```python
from build123d import *

# Parameters (mm, degrees)
ESBO_O1_W                = 53
ESBO_O1_H                = 53
RESSALTO_EXTRUS_O1_DEPTH = 3
ESBO_O3_R                = 1.3
ESBO_O3_W                = 1.2
ESBO_O3_H                = 10
CORTE_EXTRUS_O1_DEPTH    = 38.596542394
ESBO_O4_W                = 1.55
ESBO_O4_H                = 7.65
ESBO_O4_W_2              = 7.65
ESBO_O4_H_2              = 1.55
CORTE_EXTRUS_O2_DEPTH    = 10
FILETE1_R                = 15
ESBO_O5_R                = 1
CORTE_EXTRUS_O3_DEPTH    = 38.596542394


with BuildPart() as part:
    # Esboço1 → Ressalto-extrusão1 (new body)
    with BuildSketch(Plane(origin=(0, 0, 0), x_dir=(1, 0, 0), z_dir=(0, 1, 0))):
        Rectangle(ESBO_O1_W, ESBO_O1_H)
    extrude(amount=RESSALTO_EXTRUS_O1_DEPTH)

    # Esboço3 → Corte-extrusão1 (cut, through all)
    with BuildSketch(Plane(origin=(0, 3, 0), x_dir=(1, 0, 0), z_dir=(0, 1, 0))):
        with Locations(Location((0, 0, 0), (0, 0, 270))):
            Circle(ESBO_O3_R)
        with Locations((-4.4, 0)):
            Rectangle(ESBO_O3_W, ESBO_O3_H)
        with Locations((4.4, 0)):
            Rectangle(ESBO_O3_W, ESBO_O3_H)
    extrude(amount=-CORTE_EXTRUS_O1_DEPTH, mode=Mode.SUBTRACT)

    # Esboço4 → Corte-extrusão2 (cut)
    with BuildSketch(Plane(origin=(0, 3, 0), x_dir=(-1, 0, 0), z_dir=(0, 1, 0))):
        with Locations((-7.725, -9.675)):
            Rectangle(ESBO_O4_W, ESBO_O4_H)
        with Locations((-9.675, 7.725)):
            Rectangle(ESBO_O4_W_2, ESBO_O4_H_2)
        with Locations((7.725, 9.675)):
            Rectangle(ESBO_O4_W, ESBO_O4_H)
        with Locations((9.675, -7.725)):
            Rectangle(ESBO_O4_W_2, ESBO_O4_H_2)
    extrude(amount=-CORTE_EXTRUS_O2_DEPTH, mode=Mode.SUBTRACT)

    # Filete1
    filete1_edges = [part.edges().sort_by_distance(p)[0] for p in [
        (26.5, 1.5, 26.5),
        (-26.5, 1.5, 26.5),
        (-26.5, 1.5, -26.5),
        (26.5, 1.5, -26.5),
    ]]
    fillet(filete1_edges, radius=FILETE1_R)

    # Esboço5 → Corte-extrusão3 (cut, through all)
    with BuildSketch(Plane(origin=(0, 3, 0), x_dir=(1, 0, 0), z_dir=(0, 1, 0))):
        with Locations(Location((-15.742640687, -21.399494937, 0), (0, 0, 270))):
            Circle(ESBO_O5_R)
        with Locations(Location((15.742640687, 21.399494937, 0), (0, 0, 270))):
            Circle(ESBO_O5_R)
        with BuildLine():
            Line((19.566648228, -3.32990767), (14.283511733, -3.32990767))
            ThreePointArc((14.283511733, -3.32990767), (10.953604064, 0), (14.283511733, 3.32990767))
            Line((14.283511733, 3.32990767), (19.566648228, 3.32990767))
            ThreePointArc((19.566648228, 3.32990767), (22.896555897, 0), (19.566648228, -3.32990767))
        make_face()
        with BuildLine():
            Line((-3.32990767, -19.566648228), (-3.32990767, -14.283511733))
            ThreePointArc((-3.32990767, -14.283511733), (0, -10.953604064), (3.32990767, -14.283511733))
            Line((3.32990767, -14.283511733), (3.32990767, -19.566648228))
            ThreePointArc((3.32990767, -19.566648228), (0, -22.896555897), (-3.32990767, -19.566648228))
        make_face()
        with BuildLine():
            Line((-19.566648228, 3.32990767), (-14.283511733, 3.32990767))
            ThreePointArc((-14.283511733, 3.32990767), (-10.953604064, 0), (-14.283511733, -3.32990767))
            Line((-14.283511733, -3.32990767), (-19.566648228, -3.32990767))
            ThreePointArc((-19.566648228, -3.32990767), (-22.896555897, 0), (-19.566648228, 3.32990767))
        make_face()
        with BuildLine():
            Line((3.32990767, 19.566648228), (3.32990767, 14.283511733))
            ThreePointArc((3.32990767, 14.283511733), (0, 10.953604064), (-3.32990767, 14.283511733))
            Line((-3.32990767, 14.283511733), (-3.32990767, 19.566648228))
            ThreePointArc((-3.32990767, 19.566648228), (0, 22.896555897), (3.32990767, 19.566648228))
        make_face()
    extrude(amount=-CORTE_EXTRUS_O3_DEPTH, mode=Mode.SUBTRACT)


solid = part.part
```
Input: part model. Units: mm. Frame: model coordinates. Round coordinates to 2 decimals unless told otherwise and drop trailing zeros. Loops run counter-clockwise (first coordinate to the right, second up) from the corner with the lowest first, then second, coordinate; pieces in that order, holes last. Notation, with made-up numbers: M 13.5,26.5 L 54.5,26.5 A20 ccw 54.5,42.5 Z; hole C 12,-2 d2. An arc over 180 degrees is marked long. Answer in a Markdown table with one row per item. Add a question column.
1. Contact query for flat-ended pins moving along their axis: pin 1 (0.9 mm diameter, centred on x = -17.5, y = 1.5, fed in from +Z); pin 2 (1.5 mm diameter, centred on x = -17, y = 2, fed in from -Z); pin 3 (1.5 mm diameter, centred on y = 2, z = -18, fed in from +X). Output: stop coordinate, or through.
2. Mould query, pull axis X, two halves, no side actions, for faces 1 (the face through (-8, 2, 13.5)), 2 (the face through (0, 1, 26.5)), 3 (the face through (21.99, 1.52, -22.22)), 4 (the face through (-22.22, 1.52, -21.99)). Classes: released by +X, released by -X, zero draft, split by the parting line, or undercut.
3. Section C-C (y = 2.35). Give the number of separate pieces and of enclosed holes in the cut face, and give its area (3 significant figures).
4. Section B-B (x = 0). Output: boundary loops of the cut face in (y, z).
5. Ray query, probe 1 along X at (y, z) = (2.5, 0); probe 2 along Z at (x, y) = (-6, 2.45); probe 3 along X at (y, z) = (0.4, 12). Return the intervals inside material, ascending.
6. Section A-A (z = 0). Output: boundary loops of the cut face in (x, y), and give its area (3 significant figures).
Values follow:
| question | item | result |
|---|---|---|
| 1 | pin 1 | z = 25.44 |
| 1 | pin 2 | z = -25.73 |
| 1 | pin 3 | x = 25.35 |
| 2 | face 1 | undercut |
| 2 | face 2 | zero draft |
| 2 | face 3 | released by +X |
| 2 | face 4 | released by -X |
| 3 | separate pieces | 1 |
| 3 | enclosed holes | 13 |
| 3 | area | 2,250 mm^2 |
| 4 | outline | M 0,-26.5 L 3,-26.5 L 3,-22.9 L 0,-22.9 Z; M 0,-10.95 L 3,-10.95 L 3,-1.3 L 0,-1.3 Z; M 0,1.3 L 3,1.3 L 3,10.95 L 0,10.95 Z; M 0,22.9 L 3,22.9 L 3,26.5 L 0,26.5 Z |
| 5 | probe 1 | -26.5 to -22.9, -10.95 to -5, -3.8 to -1.3, 1.3 to 3.8, 5 to 10.95, 22.9 to 26.5 |
| 5 | probe 2 | -26.5 to -8.5, -6.95 to 26.5 |
| 5 | probe 3 | -26.49 to -8.5, -6.95 to -2.42, 2.42 to 26.49 |
| 6 | outline | M -26.5,0 L -22.9,0 L -22.9,3 L -26.5,3 Z; M -10.95,0 L -5,0 L -5,3 L -10.95,3 Z; M -3.8,0 L -1.3,0 L -1.3,3 L -3.8,3 Z; M 1.3,0 L 3.8,0 L 3.8,3 L 1.3,3 Z; M 5,0 L 10.95,0 L 10.95,3 L 5,3 Z; M 22.9,0 L 26.5,0 L 26.5,3 L 22.9,3 Z |
| 6 | area | 72.3 mm^2 |
